Check sheet for the modelled part. Datum: model origin and axes. Units: mm. A direction names the side the tool comes from. Coordinates: 2 decimals unless noted, no trailing zeros. Order: outer loops, then holes, each group sorted by start corner. A loop starts at its lowest first (then second) coordinate and runs counter-clockwise, first axis right, second up.
from build123d import *

# Parameters (mm, degrees)
SKETCH_1_W          = 134
SKETCH_1_H          = 73
SKETCH_1_R          = 2
SKETCH_1_W_2        = 30
SKETCH_1_H_2        = 30
EXTRUDE_1_DEPTH     = 2
SKETCH_2_W          = 34
SKETCH_2_H          = 34
SKETCH_2_W_2        = 30
SKETCH_2_H_2        = 30
EXTRUDE_2_DEPTH     = 20
SKETCH_3_W          = 34
SKETCH_3_H          = 2
EXTRUDE_4_DEPTH     = 13
EXTRUDE_5_DEPTH     = 2
EXTRUDE_6_DEPTH     = 2
EXTRUDE_8_DEPTH     = 10
EXTRUDE_9_DEPTH     = 10
SKETCH_9_R          = 2
CUT_EXTRUDE_1_DEPTH = 2


with BuildPart() as part:
    # 草图1 → 凸台-拉伸1 (new body)
    with BuildSketch(Plane(origin=(0, 0, 0), x_dir=(1, 0, 0), z_dir=(0, 1, 0))):
        with Locations((-9.171149658, 5.449528879)):
            Rectangle(SKETCH_1_W, SKETCH_1_H)
        with Locations(Location((-73.171149658, 3.949528879, 0), (0, 0, 270))):
            Circle(SKETCH_1_R, mode=Mode.SUBTRACT)
        with Locations(Location((54.828850342, 3.949528879, 0), (0, 0, 270))):
            Circle(SKETCH_1_R, mode=Mode.SUBTRACT)
        with Locations((11.799460463, 5.560834735)):
            Rectangle(SKETCH_1_W_2, SKETCH_1_H_2, mode=Mode.SUBTRACT)
    extrude(amount=EXTRUDE_1_DEPTH)

    # 草图2 → 凸台-拉伸2 (add)
    with BuildSketch(Plane(origin=(0, 2, 0), x_dir=(1, 0, 0), z_dir=(0, 1, 0))):
        with Locations((11.799460463, 5.560834735)):
            Rectangle(SKETCH_2_W, SKETCH_2_H)
        with Locations((11.799460463, 5.560834735)):
            Rectangle(SKETCH_2_W_2, SKETCH_2_H_2, mode=Mode.SUBTRACT)
    extrude(amount=EXTRUDE_2_DEPTH)

    # 草图3 → 凸台-拉伸4 (add)
    with BuildSketch(Plane(origin=(0, 22, 0), x_dir=(1, 0, 0), z_dir=(0, 1, 0))):
        with Locations((11.799460463, 21.560834735)):
            Rectangle(SKETCH_3_W, SKETCH_3_H)
    extrude(amount=EXTRUDE_4_DEPTH)

    # 草图5 → 凸台-拉伸5 (add)
    with BuildSketch(Plane(origin=(28.799460463, 0, 0), x_dir=(0, 0, -1), z_dir=(1, 0, 0))):
        Polygon((-11.439165265, 22), (20.560834735, 22), (20.560834735, 35), align=None)
    extrude(amount=-EXTRUDE_5_DEPTH)

    # 草图6 → 凸台-拉伸6 (add)
    with BuildSketch(Plane.ZY.offset(5.200539537)):
        Polygon((-20.560834735, 35), (-20.560834735, 22), (11.439165265, 22), align=None)
    extrude(amount=-EXTRUDE_6_DEPTH)

    # 草图8 → 凸台-拉伸8 (add)
    with BuildSketch(Plane.ZY.offset(5.200539537)):
        Polygon((11.439165265, 22), (11.439165265, 20.001570324), (-20.560834735, 32.989316021), (-20.560834735, 35), align=None)
    extrude(amount=EXTRUDE_8_DEPTH)

    # 草图7 → 凸台-拉伸9 (add)
    with BuildSketch(Plane(origin=(28.799460463, 0, 0), x_dir=(0, 0, -1), z_dir=(1, 0, 0))):
        Polygon((-11.439165265, 22), (20.560834735, 35), (20.560834735, 32.997882157), (-11.439165265, 19.836435038), align=None)
    extrude(amount=EXTRUDE_9_DEPTH)

    # 草图9 → 切除-拉伸1 (cut)
    with BuildSketch(Plane(origin=(0, 22.872332565, 9.291885105), x_dir=(1, 0, 0), z_dir=(0, 0.9264665771223091, 0.3763770469559383))):
        with Locations(Location((-10.200539537, 17.222122823, 0), (0, 0, 270))):
            Circle(SKETCH_9_R)
        with Locations(Location((33.799460463, 17.222122823, 0), (0, 0, 270))):
            Circle(SKETCH_9_R)
    extrude(amount=-CUT_EXTRUDE_1_DEPTH, mode=Mode.SUBTRACT)


solid = part.part
(1) Release check for a two-part mould opening along Z. For faces 1 (the flat face through (11, 12, 11.439)), 2 (the cylindrical face through (-8.514, 28.1, -6.013)), 3 (the flat face through (-15.201, 27, -4)), 4 (the flat face through (26.799, 14, -8)) record: +Z half, -Z half, draft (parallel to the pull), parting line (faces both ways), or undercut.
Filled in:
face 1: +Z half
face 2: undercut
face 3: draft
face 4: undercut
(2) Cross-section at A-A (x = -6.5). Enter the section's corners in (y, z), and give its area (3 significant figures).
Filled in:
outline: (0, -41.95) - (2, -41.95) - (2, 31.05) - (0, 31.05) - close; (20, 11.44) - (32.99, -20.56) - (35, -20.56) - (22, 11.44) - close
area: 210 mm2
(3) Thickness scan on probe 1 along X at (y, z) = (14.5, -8); probe 2 along X at (y, z) = (33, -20); probe 3 along Y at (x, z) = (-16, 0). Record the ranges inside material, lowest first.
Filled in:
probe 1: x = -5.2 to -3.2, 26.8 to 28.8
probe 2: x = -15.2 to -3.2, 26.8 to 38.8
probe 3: y = 0 to 2
(4) Go/stop test with flat-tipped pins: P1, Ø0.6, axis at x = 14, z = 10, coming from the +Y side; P2, Ø3, axis at x = -73.17, z = -3.95, coming from the +Y side; P3, Ø16, axis at y = 14.5, z = -6.5, coming from the -X side; P4, Ø10, axis at x = 17.5, y = 16, coming from the +Z side. Record where each tip stops, or that it passes through.
Filled in:
P1: stops at y = 22
P2: passes through
P3: stops at x = -5.2
P4: stops at z = 11.44
(5) Cross-section at C-C (z = 1). Enter the section's corners in (x, y).
Filled in:
outline: (-76.17, 0) - (-3.2, 0) - (-3.2, 26.24) - (-15.2, 26.24) - (-15.2, 24.24) - (-5.2, 24.24) - (-5.2, 2) - (-76.17, 2) - close; (26.8, 0) - (57.83, 0) - (57.83, 2) - (28.8, 2) - (28.8, 24.13) - (38.8, 24.13) - (38.8, 26.24) - (26.8, 26.24) - close
(6) Cross-section at B-B (y = 11). Enter the section's corners in (x, z).
Filled in:
outline: (-5.2, -22.56) - (28.8, -22.56) - (28.8, 11.44) - (-5.2, 11.44) - close; hole (-3.2, -20.56) - (26.8, -20.56) - (26.8, 9.44) - (-3.2, 9.44) - close
(7) Tool access check on faces 5 (the flat face through (28.799, 15, -5)), 6 (the flat face through (38.799, 27, -5)), 7 (the flat face through (-10.131, 26.405, -4.337)). Record the directions out of +Z, -Z, +X, -X, +Y, -Y that give a thin tool (end or side, any length) a straight path to the whole face; none if there is none.
Filled in:
face 5: -Z, +X
face 6: +Z, -Z, +X, +Y
face 7: -Z, -X
(8) Cross-section at D-D (x = 23). Enter the section's corners in (y, z).
Filled in:
outline: (0, -41.95) - (2, -41.95) - (2, -22.56) - (35, -22.56) - (35, -20.56) - (0, -20.56) - close; (0, 9.44) - (22, 9.44) - (22, 11.44) - (2, 11.44) - (2, 31.05) - (0, 31.05) - close
